Print and shaded views of the part. All mm, measured from the part's lowest x, y and z. A direction names the side the tool comes from. Round coordinates to 2 decimals unless told otherwise and drop trailing zeros. Order: outer loops, then holes, each group sorted by start corner. A loop starts at its lowest first (then second) coordinate and runs counter-clockwise, first axis right, second up. Notation, with made-up numbers: (11.25, 57) - (25.25, 57) arc R29 cw to (25.25, 90) - close; hole circle Ø5 at (-28, -31). An arc over 180 degrees is marked (long way). Write item = value, one per line.
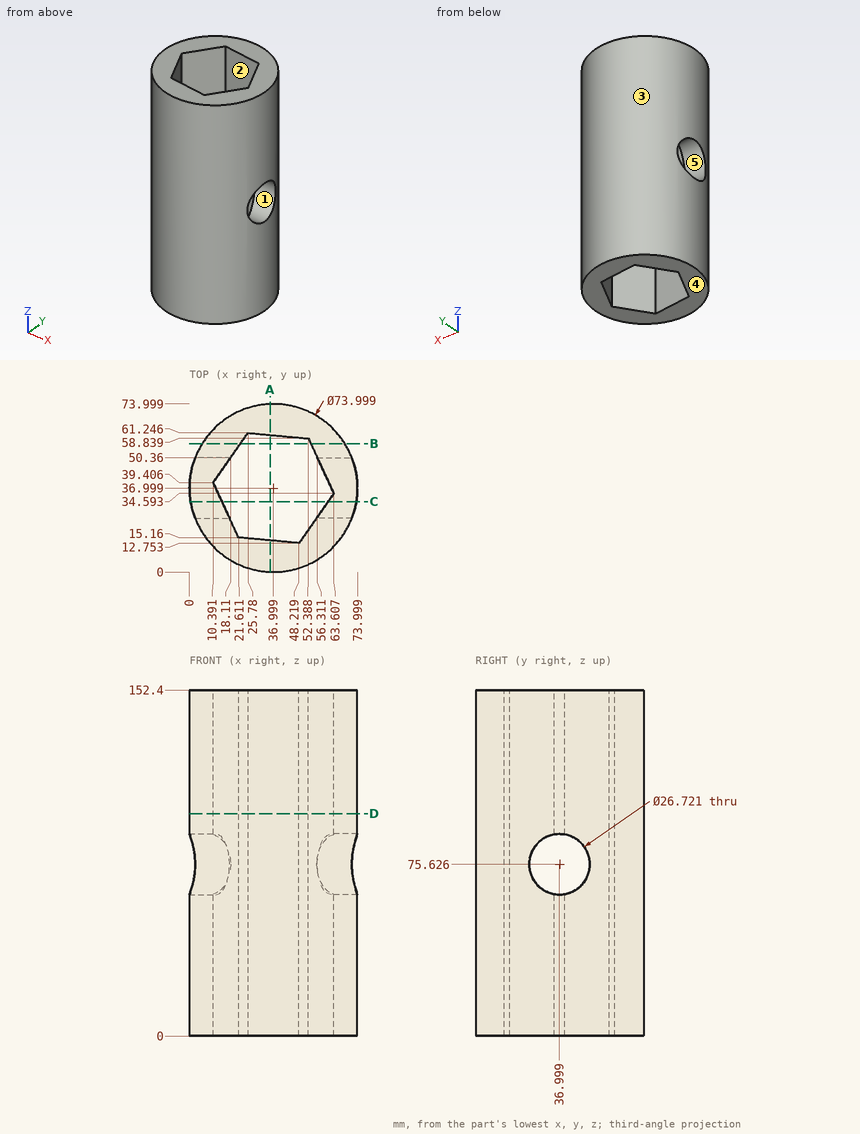
(1) Band-saw the part on D-D on z = 98. List the corners of the cut face in (x, y) (1 decimal).
Solved:
outline = circle Ø74 at (37, 37); hole (10.4, 39.4) - (21.6, 15.2) - (48.2, 12.8) - (63.6, 34.6) - (52.4, 58.8) - (25.8, 61.2) - close
(2) Probe line 1 along Y through (x, z) = (44.5, 20); line 2 along X through (y, z) = (19.5, 84) (1 decimal); line 3 along Y through (x, z) = (37, 69). List the from-to ranges inside material, lowest first.
Solved:
line_1 = 0.77 to 13.09, 59.55 to 73.23
line_2 = 4.4 to 19.6, 53 to 69.6
line_3 = 0 to 13.77, 60.23 to 74
(3) Tool access for the marked faces 1 and 2: list every direction of +Z, -Z, +X, -X, +Y, -Y with a clear straight run to the whole face (end or side of a thin tool).
Solved:
face_1 = +X, -X
face_2 = +Z, -Z
(4) Band-saw the part on A-A on x = 35.5. List the corners of the cut face in (y, z).
Solved:
outline = (0.03, 0) - (13.9, 0) - (13.9, 152.4) - (0.03, 152.4) - close; (60.37, 0) - (73.97, 0) - (73.97, 152.4) - (60.37, 152.4) - close
(5) Band-saw the part on B-B on y = 56.5. List the corners of the cut face in (x, z) (1 decimal).
Solved:
outline = (5.6, 0) - (22.4, 0) - (22.4, 152.4) - (5.6, 152.4) - close; (53.5, 0) - (68.4, 0) - (68.4, 152.4) - (53.5, 152.4) - close
(6) Band-saw the part on C-C on y = 31. List the corners of the cut face in (x, z), plus the area to 3 significant figures.
Solved:
outline = (0.49, 0) - (14.28, 0) - (14.28, 63.69) - (0.49, 63.69) - close; (0.49, 87.56) - (14.28, 87.56) - (14.28, 152.4) - (0.49, 152.4) - close; (61.08, 0) - (73.51, 0) - (73.51, 63.69) - (61.08, 63.69) - close; (61.08, 87.56) - (73.51, 87.56) - (73.51, 152.4) - (61.08, 152.4) - close
area = 3,370 mm²
(7) Drop flat-ended pins along their axis: pin 1 (12 mm diameter, centred on x = 32.5, z = 82.5, fed in from +Y); pin 2 (21.5 mm diameter, centred on y = 37, z = 75.63, fed in from -X); pin 3 (12 mm diameter, centred on y = 24.5, z = 24, fed in from -X) (1 decimal); pin 4 (5 mm diameter, centred on y = 50.5, z = 94, fed in from +X) (1 decimal). Give the stop position or say it passes through.
Solved:
pin_1 = 74
pin_2 = through
pin_3 = 0.6
pin_4 = 72.3
(8) Pull direction Y, two halves, no side cores. Call the marked faces 3, 4 and 5: released by +Y, released by -Y, zero draft, split by the parting line, or undercut.
Solved:
face_3 = split by the parting line
face_4 = zero draft
face_5 = undercut
